The listing builds one solid part. Answer for the finished solid, in the listing's coordinates (mm). A direction names the side the tool comes from. Give positions to 0.01 mm unless a question says otherwise; leave off trailing zeros. Loops run counter-clockwise (first coordinate to the right, second up) from the corner with the lowest first, then second, coordinate; pieces in that order, holes last.
Item 1: Each of these flat-tipped pins is pushed along its axis until it touches: pin 1 Ø1.3 at (x, y) = (-13.5, -4.5) entering from -Z; pin 2 Ø0.9 at (y, z) = (-86.5, 2) entering from -X; pin 3 Ø2 at (x, y) = (5.59, -75) entering from -Z; pin 4 Ø5 at (x, y) = (12.88, -5.01) entering from -Z. Where does it stop, or does it pass through?
Item 2: Section A-A, the plane x = 1 is taken. Give the vertices of the cut face in (y, z).
Item 3: Section B-B, the plane y = -33.5 is taken. Give the vertices of the cut face in (x, z).
Item 4: Section D-D, the plane y = -10 is taken. Give the vertices of the cut face in (x, z).
Item 5: Section C-C, the plane z = 0.9 is taken. Give the number of separate pieces and of enclosed holes in the cut face, and give its area (3 significant figures).
Item 6: The mould has two halves that part along X. Classify faces 4 (the face through (-13.764, -4.201, 2.507)), 5 (the face through (0, -35, 0)), 6 (the face through (13.483, -52.14, 1.479)): pulls with the +X half, pulls with the -X half, needs draft (parallel to the pull), parting line crosses it, or undercut.
Item 7: Consider line 1 along X through (y, z) = (-25.5, 2.15); line 2 along X through (y, z) = (-63, 1.3) (3 decimals); line 3 along X through (y, z) = (-12, 0.8). Determine where each line is inside the solid, lowest interval first.
Item 8: A tool of negligible diameter and unlimited length cuts with its end or side. For faces 1 (the face through (0, -100, 1)), 2 (the face through (-7, -76, 2)), 3 (the face through (-4, -70, 2)), from which of +Z, -Z, +X, -X, +Y, -Y can it reach the whole face along a straight path? Write none if from no direction.
from build123d import *

# Parameters (mm, degrees)
EXTRUDE_1_DEPTH              = 3
CUT_EXTRUDE_1_REACH          = 104.025
SKETCH_2_W                   = 5
SKETCH_2_H                   = 10
HOLE_WIZARD_M2_1_D           = 2.4
HOLE_WIZARD_M2_1_CBORE_D     = 4.4
HOLE_WIZARD_M2_1_CBORE_DEPTH = 2
CUT_EXTRUDE_2_REACH          = 104.025
SKETCH_5_R                   = 4
HOLE_WIZARD_M2_2_D           = 2.4
HOLE_WIZARD_M2_2_CBORE_D     = 4.4
HOLE_WIZARD_M2_2_CBORE_DEPTH = 2
HOLE_WIZARD_M2_3_D           = 2.4
HOLE_WIZARD_M2_3_CBORE_D     = 4.4
HOLE_WIZARD_M2_3_CBORE_DEPTH = 2
CUT_EXTRUDE_3_DEPTH          = 3
HOLE_WIZARD_M2_5_D           = 2.4
HOLE_WIZARD_M2_5_CBORE_D     = 4.4
HOLE_WIZARD_M2_5_CBORE_DEPTH = 2
HOLE_WIZARD_M2_6_D           = 2.4
HOLE_WIZARD_M2_6_CBORE_D     = 4.4
HOLE_WIZARD_M2_6_CBORE_DEPTH = 2
CUT_EXTRUDE_4_DEPTH          = 10


with BuildPart() as part:
    # 草图1 → 凸台-拉伸1 (new body)
    with BuildSketch(Plane.XY):
        Polygon((20, 5), (20, 45), (19.258297735, 54.944681764), (13.241702265, 95.055318236), (7.5, 100), (-7.5, 100), (-13.241702265, 95.055318236), (-19.258297735, 54.944681764), (-20, 45), (-20, 5), (-19.379826327, -4.961389384), (-7.748069469, -98.015444247), (-5.5, -100), (5.5, -100), (7.748069469, -98.015444247), (19.379826327, -4.961389384), align=None)
    extrude(amount=EXTRUDE_1_DEPTH)

    # 草图2 → 切除-拉伸1 (cut, up to next)
    with BuildSketch(Plane.XY.offset(3), mode=Mode.PRIVATE) as cut_extrude_1_sk1:
        Polygon((10, -5), (-10, -5), (0, -22.320508076), align=None)
    cut_extrude_1_tool1 = extrude(cut_extrude_1_sk1.sketch, amount=-CUT_EXTRUDE_1_REACH, mode=Mode.PRIVATE) & part.part
    # 草图2 → 切除-拉伸1 (cut, up to next)
    with BuildSketch(Plane.XY.offset(3), mode=Mode.PRIVATE) as cut_extrude_1_sk2:
        Polygon((6.211088907, -70), (13.938881842, -8.177656525), (2.5, -27.990381057), (2.5, -70), align=None)
    cut_extrude_1_tool2 = extrude(cut_extrude_1_sk2.sketch, amount=-CUT_EXTRUDE_1_REACH, mode=Mode.PRIVATE) & part.part
    # 草图2 → 切除-拉伸1 (cut, up to next)
    with BuildSketch(Plane.XY.offset(3), mode=Mode.PRIVATE) as cut_extrude_1_sk3:
        Polygon((-13.938881842, -8.177656525), (-2.5, -27.990381057), (-2.5, -70), (-6.211088907, -70), align=None)
    cut_extrude_1_tool3 = extrude(cut_extrude_1_sk3.sketch, amount=-CUT_EXTRUDE_1_REACH, mode=Mode.PRIVATE) & part.part
    # 草图2 → 切除-拉伸1 (cut, up to next)
    with BuildSketch(Plane.XY.offset(3), mode=Mode.PRIVATE) as cut_extrude_1_sk4:
        with Locations((0, -85)):
            Rectangle(SKETCH_2_W, SKETCH_2_H)
    cut_extrude_1_tool4 = extrude(cut_extrude_1_sk4.sketch, amount=-CUT_EXTRUDE_1_REACH, mode=Mode.PRIVATE) & part.part
    add(cut_extrude_1_tool1.solids().sort_by_distance((0, -10.773503, 3))[0], mode=Mode.SUBTRACT)
    add(cut_extrude_1_tool2.solids().sort_by_distance((6.712708, -39.914502, 3))[0], mode=Mode.SUBTRACT)
    add(cut_extrude_1_tool3.solids().sort_by_distance((-6.712708, -39.914502, 3))[0], mode=Mode.SUBTRACT)
    add(cut_extrude_1_tool4.solids().sort_by_distance((0, -85, 3))[0], mode=Mode.SUBTRACT)

    # M2 凹头盖螺钉的柱形沉头孔1 (through all)
    with Locations(Plane(origin=(5.586088907, -75, 0), x_dir=(-1, 0, 0), z_dir=(0, 0, -1))):
        with Locations((0, 0), (11.172177814, 0)):
            CounterBoreHole(HOLE_WIZARD_M2_1_D / 2, HOLE_WIZARD_M2_1_CBORE_D / 2, HOLE_WIZARD_M2_1_CBORE_DEPTH)

    # 草图5 → 切除-拉伸2 (cut, up to next)
    with BuildSketch(Plane(origin=(0, 0, 0), x_dir=(-1, 0, 0), z_dir=(0, 0, -1)), mode=Mode.PRIVATE) as cut_extrude_2_sk1:
        with Locations((0, 25)):
            Circle(SKETCH_5_R)
    cut_extrude_2_tool1 = extrude(cut_extrude_2_sk1.sketch, amount=-CUT_EXTRUDE_2_REACH, mode=Mode.PRIVATE) & part.part
    add(cut_extrude_2_tool1.solids().sort_by_distance((0, 25, 0))[0], mode=Mode.SUBTRACT)

    # M2 凹头盖螺钉的柱形沉头孔2 (through all)
    with Locations(Plane(origin=(8, 25, 0), x_dir=(-1, 0, 0), z_dir=(0, 0, -1))):
        with Locations((0, 0), (8, 8), (16, 0), (8, -8)):
            CounterBoreHole(HOLE_WIZARD_M2_2_D / 2, HOLE_WIZARD_M2_2_CBORE_D / 2, HOLE_WIZARD_M2_2_CBORE_DEPTH)

    # M2 凹头盖螺钉的柱形沉头孔3 (through all)
    with Locations(Plane(origin=(12.880020708, -5.011657807, 0), x_dir=(-1, 0, 0), z_dir=(0, 0, -1))):
        with Locations((0, 0), (25.760041416, 0)):
            CounterBoreHole(HOLE_WIZARD_M2_3_D / 2, HOLE_WIZARD_M2_3_CBORE_D / 2, HOLE_WIZARD_M2_3_CBORE_DEPTH)

    # 草图10 → 切除-拉伸3 (cut)
    with BuildSketch(Plane(origin=(0, 0, 0), x_dir=(-1, 0, 0), z_dir=(0, 0, -1))):
        Polygon((-14.016935065, 56.180852205), (-10.679274874, 78.431920145), (-8.411945476, 80.068406675), (-4.470648492, 79.385634325), (-2.5, 77.04424815), (-2.5, 56.2029795), (-4.5, 54.2029795), (-12.313615971, 54.2029795), align=None)
        Polygon((-9.344020618, 87.333615184), (-8.2970205, 94.313615971), (0, 94.313615971), (8.2970205, 94.313615971), (9.344020618, 87.333615184), (7.670053032, 85.014356303), (0, 83.685631227), (-7.670053032, 85.014356303), align=None)
        Polygon((4.5, 54.2029795), (12.313615971, 54.2029795), (14.016935065, 56.180852205), (10.679274874, 78.431920145), (8.411945476, 80.068406675), (4.470648492, 79.385634325), (2.5, 77.04424815), (2.5, 56.2029795), align=None)
    extrude(amount=-CUT_EXTRUDE_3_DEPTH, mode=Mode.SUBTRACT)

    # M2 凹头盖螺钉的柱形沉头孔5 (through all)
    with Locations(Plane(origin=(0, 79.840052868, 0), x_dir=(-1, 0, 0), z_dir=(0, 0, -1))):
        with Locations((0, 0)):
            CounterBoreHole(HOLE_WIZARD_M2_5_D / 2, HOLE_WIZARD_M2_5_CBORE_D / 2, HOLE_WIZARD_M2_5_CBORE_DEPTH)

    # M2 凹头盖螺钉的柱形沉头孔6 (through all)
    with Locations(Plane(origin=(12.880020708, 14.988342193, 0), x_dir=(-1, 0, 0), z_dir=(0, 0, -1))):
        with Locations((0, 0), (25.760041416, 0)):
            CounterBoreHole(HOLE_WIZARD_M2_6_D / 2, HOLE_WIZARD_M2_6_CBORE_D / 2, HOLE_WIZARD_M2_6_CBORE_DEPTH)

    # 草图17 → 切除-拉伸4 (cut)
    with BuildSketch(Plane(origin=(0, 0, 0), x_dir=(-1, 0, 0), z_dir=(0, 0, -1))):
        Polygon((-20, 5), (20, 5), (20, 99.998273705), (7.5, 100), (-7.5, 100), (-20, 99.998273705), align=None)
    extrude(amount=-CUT_EXTRUDE_4_DEPTH, mode=Mode.SUBTRACT)


solid = part.part
Worked answers:
1. pin 1: stops at z = 2
1. pin 2: stops at x = -9.24
1. pin 3: passes through
1. pin 4: stops at z = 0
2. outline: (-100, 0) - (-90, 0) - (-90, 3) - (-100, 3) - close; (-80, 0) - (-20.59, 0) - (-20.59, 3) - (-80, 3) - close; (-5, 0) - (5, 0) - (5, 3) - (-5, 3) - close
3. outline: (-15.81, 0) - (-10.77, 0) - (-10.77, 3) - (-15.81, 3) - close; (-2.5, 0) - (2.5, 0) - (2.5, 3) - (-2.5, 3) - close; (10.77, 0) - (15.81, 0) - (15.81, 3) - (10.77, 3) - close
4. outline: (-18.75, 0) - (-13.71, 0) - (-13.71, 3) - (-18.75, 3) - close; (-12.89, 0) - (-7.11, 0) - (-7.11, 3) - (-12.89, 3) - close; (7.11, 0) - (12.89, 0) - (12.89, 3) - (7.11, 3) - close; (13.71, 0) - (18.75, 0) - (18.75, 3) - (13.71, 3) - close
5. separate pieces: 1
5. enclosed holes: 8
5. area: 1,950 mm2
6. face 4: undercut
6. face 5: needs draft
6. face 6: pulls with the +X half
7. line 1: x = -16.81 to -11.77, -3.94 to 3.94, 11.77 to 16.81
7. line 2: x = -12.125 to -7.086, -2.5 to 2.5, 7.086 to 12.125
7. line 3: x = -18.5 to -13.46, -11.73 to -5.96, 5.96 to 11.73, 13.46 to 18.5
8. face 1: +Z, -Z, +X, -X, -Y
8. face 2: -Z
8. face 3: +Z, -Z
